Build history of the part. All positions in model axes, mm. A direction names the side the tool comes from. Round coordinates to 2 decimals unless told otherwise and drop trailing zeros. Loops run counter-clockwise (first coordinate to the right, second up) from the corner with the lowest first, then second, coordinate; pieces in that order, holes last. Notation, with made-up numbers: (77, -16.5) - (127, -16.5) arc R5 cw to (127, -12.5) - close; hole circle Ø6 at (31, 12.25). An arc over 180 degrees is marked (long way). One line per question, with ' | ' between items. Start each with the question number.
from build123d import *

# Parameters (mm, degrees)
BOSS_EXTRUDE1_DEPTH = 25
SKETCH3_W           = 80
SKETCH3_H           = 80
CUT_EXTRUDE2_DEPTH  = 26


with BuildPart() as part:
    # Sketch1 → Boss-Extrude1 (new body)
    with BuildSketch(Plane.XY):
        Polygon((50, 0), (185, 0), (185, 80), (515, 80), (515, 0), (650, 0), (627.623420178, 320), (72.376579822, 320), align=None)
    extrude(amount=BOSS_EXTRUDE1_DEPTH)

    # Sketch3 → Cut-Extrude2 (cut, through all)
    with BuildSketch(Plane.XY.offset(25)):
        with Locations((145, 40)):
            Rectangle(SKETCH3_W, SKETCH3_H)
        with Locations((555, 40)):
            Rectangle(SKETCH3_W, SKETCH3_H)
    extrude(amount=-CUT_EXTRUDE2_DEPTH, mode=Mode.SUBTRACT)


solid = part.part
1) Saw through at A-A on z = 16. Write the cut outline in (x, y), and give its area (3 significant figures).
2) Saw through at C-C on y = 222.5. Write the cut outline in (x, z), and give its area (3 significant figures).
3) Saw through at B-B on x = 532. Write the cut outline in (y, z).
4) Wall check: line 1 (Y direction, x = 480, z = 6.75); line 2 (X direction, y = 66.5, z = 15.5); line 3 (X direction, y = 184.5, z = 7.75). Give the ranges that are in metal, low to high. Write a range as [from, to].
5) Two-plate mould, pull along X, no slides. Class faces 3 (the flat face through (595, 39, 13)), 4 (the flat face through (638.97, 157.76, 12.32)), 5 (the flat face through (105, 39, 13)), 6 (the flat face through (346, 198, 25)): +X half, -X half, draft (parallel to the pull), parting line (faces both ways), or undercut.
6) Drop flat-ended pins along their axis: pin 1 (12.5 mm diameter, centred on x = 423.5, z = 7.5, fed in from -Y); pin 2 (12 mm diameter, centred on y = 114.5, z = 10, fed in from -X). Give the stop position or say it passes through.
7) Tool access for faces 1 (the flat face through (347, 80, 13)), 2 (the flat face through (77, 0, 12)): list every direction of +Z, -Z, +X, -X, +Y, -Y with a clear straight run to the whole face (end or side of a thin tool).
Answer key:
1) outline: (50, 0) - (105, 0) - (105, 80) - (595, 80) - (595, 0) - (650, 0) - (627.62, 320) - (72.38, 320) - close | area: 146,000 mm²
2) outline: (65.56, 0) - (634.44, 0) - (634.44, 25) - (65.56, 25) - close | area: 14,200 mm²
3) outline: (80, 0) - (320, 0) - (320, 25) - (80, 25) - close
4) line 1: [80, 320] | line 2: [54.65, 105], [595, 645.35] | line 3: [62.9, 637.1]
5) face 3: undercut | face 4: +X half | face 5: undercut | face 6: draft
6) pin 1: y = 80 | pin 2: x = 57.59
7) face 1: +Z, -Z, -Y | face 2: +Z, -Z, +X, -X, -Y
